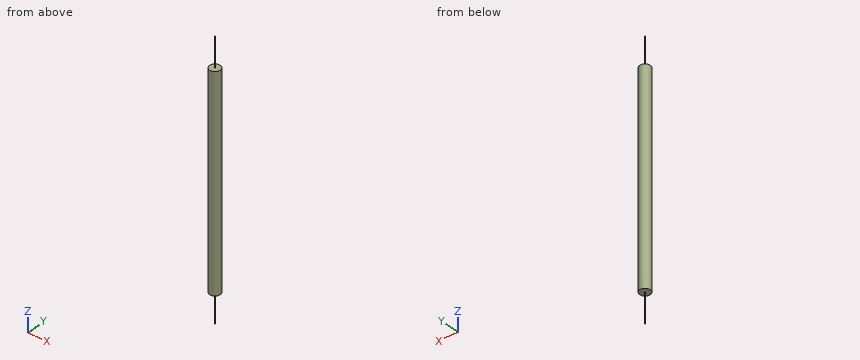
```python
from build123d import *

# Parameters (mm, degrees)
SKETCH_7_R          = 5
EXTRUDE_4_DEPTH     = 200
SKETCH_8_R          = 0.5
EXTRUDE_5_DEPTH     = 28
EXTRUDE_START       = 84
SKETCH_9_R          = 0.5
EXTRUDE_6_DEPTH     = 84
SKETCH_10_R         = 0.5
CUT_EXTRUDE_1_DEPTH = 56


with BuildPart() as part:
    # 草图7 → 凸台-拉伸4 (new body)
    with BuildSketch(Plane.XY):
        Circle(SKETCH_7_R)
    extrude(amount=EXTRUDE_4_DEPTH)

    # 草图8 → 凸台-拉伸5 (add)
    with BuildSketch(Plane.XY.offset(200)):
        Circle(SKETCH_8_R)
    extrude(amount=EXTRUDE_5_DEPTH)

    # 草图9 → 凸台-拉伸6 (add)
    with BuildSketch(Plane(origin=(0, 0, 0), x_dir=(-1, 0, 0), z_dir=(0, 0, -1)).offset(EXTRUDE_START)):
        with Locations(Location((0, 0, 0), (0, 0, 180))):
            Circle(SKETCH_9_R)
    extrude(amount=-EXTRUDE_6_DEPTH)

    # 草图10 → 切除-拉伸1 (cut)
    with BuildSketch(Plane(origin=(0, 0, -84), x_dir=(-1, 0, 0), z_dir=(0, 0, -1))):
        with Locations(Location((0, 0, 0), (0, 0, 180))):
            Circle(SKETCH_10_R)
    extrude(amount=-CUT_EXTRUDE_1_DEPTH, mode=Mode.SUBTRACT)


solid = part.part
```
Geometry check sheet. Reference: the model listing, model coordinates, mm. Coordinates: 2 decimals unless noted, no trailing zeros. Write each loop counter-clockwise with the first axis right and the second up, starting at its lowest first coordinate (ties: lowest second). Pieces come first, ordered by that corner, then holes. Notation, with made-up numbers: M -38,81.5 L -22,81.5 A30 cw -22,120.5 Z; hole C 27.25,59 d2. An arc over 180 degrees is marked long. One line per item, written item: value. Start each with the question number.
(1) Scan lines: line 1 along Z through (x, y) = (4, -1.5); line 2 along X through (y, z) = (0.25, 90); line 3 along Y through (x, z) = (-3.75, 24). Record each from-to range of solid material in increasing order. Write a range as [from, to].
(2) Sectioned sample at C-C, the plane z = 33. Enter the section's corners in (x, y).
(3) Sectioned sample at A-A, the plane z = 212. Enter the section's corners in (x, y), and give its area (3 significant figures).
(4) Sectioned sample at B-B, the plane x = 3.5. Enter the section's corners in (y, z), and give its area (3 significant figures).
(5) Depth check by flat-ended pin: pin 1 (3 mm diameter, centred on y = -3, z = 137.5, fed in from +X); pin 2 (1.5 mm diameter, centred on x = -3, y = 1.5, fed in from -Z); pin 3 (4 mm diameter, centred on y = -4, z = 53, fed in from +X). Enter the tip coordinate at first touch or a pass-through.
Filled sheet:
1. line 1: [0, 200]
1. line 2: [-4.99, 4.99]
1. line 3: [-3.31, 3.31]
2. outline: C 0,0 d10
3. outline: C 0,0 d1
3. area: 0.785 mm²
4. outline: M -3.57,0 L 3.57,0 L 3.57,200 L -3.57,200 Z
4. area: 1,430 mm²
5. pin 1: x = 4.77
5. pin 2: z = 0
5. pin 3: x = 4.58
